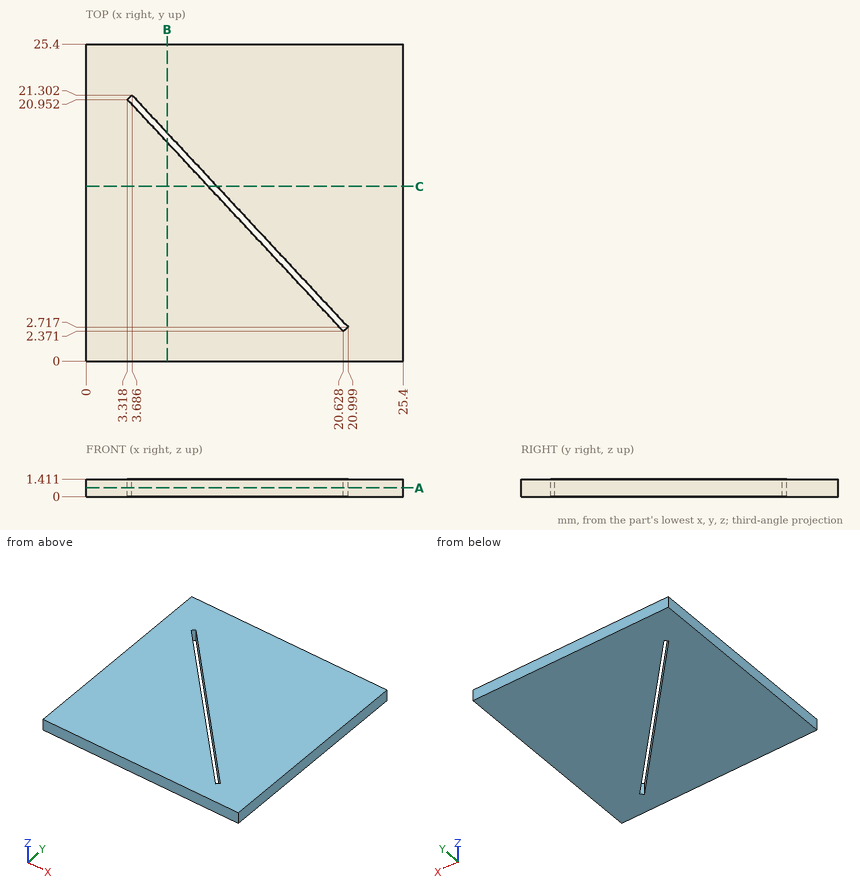
Geometry check sheet. Reference: drawing and pictorial views, mm from the part's lowest x, y, z. Round coordinates to 2 decimals unless told otherwise and drop trailing zeros. Write each loop counter-clockwise with the first axis right and the second up, starting at its lowest first coordinate (ties: lowest second). Pieces come first, ordered by that corner, then holes.
(1) Section check B-B (x = 6.5). Enter the section's corners in (y, z).
Returned:
outline: (0, 0) - (17.54, 0) - (17.54, 1.41) - (0, 1.41) - close; (18.28, 0) - (25.4, 0) - (25.4, 1.41) - (18.28, 1.41) - close
(2) Material ranges on line 1 (Y direction, x = 6.5, z = 1.2) (1 decimal); line 2 (X direction, y = 2.5, z = 0.7) (1 decimal); line 3 (Y direction, x = 7, z = 0.35) (1 decimal), recorded low to high.
Returned:
line 1: y = 0 to 17.5, 18.3 to 25.4
line 2: x = 0 to 20.5, 20.8 to 25.4
line 3: y = 0 to 17, 17.7 to 25.4
(3) Section check A-A (z = 0.7). Enter the section's corners in (x, y) (1 decimal).
Returned:
outline: (0, 0) - (25.4, 0) - (25.4, 25.4) - (0, 25.4) - close; hole (3.3, 21) - (20.6, 2.4) - (21, 2.7) - (3.7, 21.3) - close
(4) Section check C-C (y = 14). Enter the section's corners in (x, z) (1 decimal).
Returned:
outline: (0, 0) - (9.8, 0) - (9.8, 1.4) - (0, 1.4) - close; (10.5, 0) - (25.4, 0) - (25.4, 1.4) - (10.5, 1.4) - close
